Read the model definition and answer for the solid it produces. Units are mm, in the model's axes. A direction names the side the tool comes from. Coordinates: 2 decimals unless noted, no trailing zeros. Loops run counter-clockwise (first coordinate to the right, second up) from the corner with the lowest first, then second, coordinate; pieces in that order, holes last. Notation, with made-up numbers: (-26.75, 19) -> (12.25, 19) arc R26 ccw to (12.25, 50) -> close; hole circle Ø10 at (88, -33). An arc over 180 degrees is marked (long way). Answer as a JSON object with one key per item and string values. Group by question number.
1) Determine the mould class of faces 3 (the face through (10.6, -10, -3.2)), 4 (the face through (9.91, 1.73, 7.81)), 5 (the face through (15, -5, 9)) for opening direction Y: released by +Y, released by -Y, zero draft, split by the parting line, or undercut.
2) Which of the six approach directions +Z, -Z, +X, -X, +Y, -Y give full straight-line access (tool end or side, diameter ignored) to faces 1 (the face through (5, 8, -8)), 2 (the face through (0, -0.2, 8.3))?
3) Consider probe 1 along Z at (x, y) = (13.25, 0); probe 2 along Z at (x, y) = (14, 6.5); probe 3 along X at (y, z) = (-7.25, 8.75). Determine where each line is inside the solid, lowest interval first. Write a range as [from, to].
4) Flat-ended cylindrical pins translate along their axes: P1, Ø1.5, axis at x = 3, y = 4.5, coming from the -Z side; P2, Ø12, axis at x = 15, z = -9, coming from the -Y side; P3, Ø5, axis at x = 13, z = -3, coming from the +Y side. Find the tip coordinate at first contact, or state that the pin passes through.
5) Section A-A, the plane y = 0 is taken. Give the vertices of the cut face in (x, z), plus the area to 3 significant figures.
6) Section B-B, the plane x = 15.5 is taken. Give the vertices of the cut face in (y, z).
from build123d import *


with BuildPart() as part:
    # Esboço1 → Revolução1 (revolve)
    with BuildSketch(Plane.XY, mode=Mode.PRIVATE) as revolu_o1_sk:
        with BuildLine():
            Line((0, 8.05), (0, 12.7))
            Line((0, 12.7), (5, 12.7))
            Line((5, 12.7), (5, 10.5))
            ThreePointArc((5, 10.5), (5.5, 10), (6, 10.5))
            Line((6, 10.5), (15, 10.5))
            Line((15, 10.5), (15, 10))
            Line((15, 10), (20, 10))
            Line((20, 10), (20, 8))
            Line((20, 8), (0.1, 8))
            Line((0.1, 8), (0.1, 8.05))
            Line((0.1, 8.05), (0, 8.05))
        make_face()
    revolve(revolu_o1_sk.sketch.rotate(Axis((-138.925343643, 0, 0), (1, 0, 0)), 180), axis=Axis((-138.925343643, 0, 0), (1, 0, 0)))  # turned: the seam where the file's is


solid = part.part
Determined:
{
 "1": {"face 3": "split by the parting line", "face 4": "undercut", "face 5": "zero draft"},
 "2": {"face 1": "+X", "face 2": "+Z, -Z, -X, +Y, -Y"},
 "3": {"probe 1": "[-10.5, -8], [8, 10.5]", "probe 2": "[-8.25, -4.66], [4.66, 8.25]", "probe 3": "[0, 5]"},
 "4": {"P1": "z = -12.13", "P2": "y = -10.06", "P3": "y = 10.49"},
 "5": {"outline": "(0, -12.7) -> (5, -12.7) -> (5, -10.5) arc R0.5 cw to (6, -10.5) -> (15, -10.5) -> (15, -10) -> (20, -10) -> (20, -8) -> (0.1, -8) -> (0.1, -8.05) -> (0, -8.05) -> close; (0, 8.05) -> (0.1, 8.05) -> (0.1, 8) -> (20, 8) -> (20, 10) -> (15, 10) -> (15, 10.5) -> (6, 10.5) arc R0.5 cw to (5, 10.5) -> (5, 12.7) -> (0, 12.7) -> close", "area": "116 mm²"},
 "6": {"outline": "circle Ø20 at (0, 0); hole circle Ø16 at (0, 0)"}
}
